```python
from build123d import *

# Parameters (mm, degrees)
F1_R     = 6.5
F1_R_2   = 5.5
F3_DEPTH = 3
F4_DEPTH = 1.5
F5_DEPTH = 0.6
F6_DEPTH = 1
F7_DEPTH = 1
F8_DEPTH = 1


# Not quite as in the source:
# - ends of sketch curves that miss each other by under 0.0002 mm in the source are joined
# - the dataset's text gives a spline's control points without its knots; the knots are read off the source's solid


with BuildPart() as f3:
    # F1 (on Front) → F3 (new body)
    with BuildSketch(Plane.XZ):
        with Locations((1.996e-07, 0.145563783)):
            Circle(F1_R)
        with Locations((1.996e-07, 0.145563783)):
            Circle(F1_R_2, mode=Mode.SUBTRACT)
    extrude(amount=-F3_DEPTH)

    # F0 (on Front) + F1 (on Front) → F4 (join)
    with BuildSketch(Plane.XZ):
        with BuildLine():
            add(Edge.make_bspline(
                [(-1.4633628161, -3.8408698747), (-0.8618942381, -4.0797628795), (1.7775925035, -4.2725148883), (2.1266039699, -2.4883414841), (2.1792066492, -0.8570773415), (2.1261946367, 0.7652860278), (1.8591945487, 1.4152828688), (2.1073079889, 1.4090746613), (2.1070261206, 1.5973545621), (1.8482611221, 1.6571502022), (1.9106924097, 2.0013449435), (1.883292753, 2.4559971082), (1.4530608962, 2.5796008165), (1.3486705812, 2.982608362), (0.9522813685, 3.1051443516), (0.6376593936, 3.1670181532), (0.4331394013, 3.4063180529), (0.6426984155, 3.8176132891), (0.3981993423, 4.2634916825), (-0.0062082347, 4.3047771669), (-0.3006353253, 4.2313929361), (-0.6271454426, 3.9609581822), (-0.5601436399, 3.6082200906), (-0.4158755178, 3.3585569408), (-0.6804152796, 3.1141950016), (-1.0068060059, 3.1249120402), (-1.1963426018, 2.8920399235), (-1.3913162215, 2.8683333491), (-1.3804892819, 2.6236576239), (-1.7077578499, 2.7520009173), (-1.8276300328, 2.3206081403), (-1.8540486856, 2.0110635487), (-1.8641412125, 1.6986764558), (-2.1169141262, 1.6232767981), (-2.0818952059, 1.4062115725), (-1.9001690611, 1.4703026422), (-2.1146422172, 0.8809803752), (-2.0979861646, 0.2234423606), (-2.2011740498, -0.523800053), (-2.1724225003, -1.2230030424), (-2.1779022447, -2.5473945892), (-1.9120269544, -3.4285716282), (-1.7403824301, -3.7308424346), (-1.4633628161, -3.8408698747)],
                knots=[0, 0, 0, 0, 0.0614284178, 0.105210304, 0.1528188952, 0.1998934744, 0.2260159491, 0.2394622475, 0.2521789794, 0.2685961982, 0.2887254165, 0.3121716538, 0.3345624104, 0.3566054098, 0.3791085644, 0.3997521347, 0.4178904262, 0.4412373911, 0.4652934844, 0.487296569, 0.5074239254, 0.5296841222, 0.5504706917, 0.5687295132, 0.5882529988, 0.6087082105, 0.6278548545, 0.642595893, 0.6569229468, 0.674176944, 0.6961346625, 0.7176137944, 0.736576695, 0.7535032789, 0.767308469, 0.7778501968, 0.8029343179, 0.8341377518, 0.8649078271, 0.8956216456, 0.9374997946, 0.9717077879, 1, 1, 1, 1], degree=3))
        make_face()
    with BuildSketch(Plane.XZ):
        with Locations((1.996e-07, 0.145563783)):
            Circle(F1_R_2)
    extrude(amount=-F4_DEPTH)

    # F1 (on Front) + F0 (on Front) → F5 (cut)
    with BuildSketch(Plane.XZ):
        with Locations((1.996e-07, 0.145563783)):
            Circle(F1_R_2)
    with BuildSketch(Plane.XZ):
        with BuildLine():
            add(Edge.make_bspline(
                [(-1.4633628161, -3.8408698747), (-0.8618942381, -4.0797628795), (1.7775925035, -4.2725148883), (2.1266039699, -2.4883414841), (2.1792066492, -0.8570773415), (2.1261946367, 0.7652860278), (1.8591945487, 1.4152828688), (2.1073079889, 1.4090746613), (2.1070261206, 1.5973545621), (1.8482611221, 1.6571502022), (1.9106924097, 2.0013449435), (1.883292753, 2.4559971082), (1.4530608962, 2.5796008165), (1.3486705812, 2.982608362), (0.9522813685, 3.1051443516), (0.6376593936, 3.1670181532), (0.4331394013, 3.4063180529), (0.6426984155, 3.8176132891), (0.3981993423, 4.2634916825), (-0.0062082347, 4.3047771669), (-0.3006353253, 4.2313929361), (-0.6271454426, 3.9609581822), (-0.5601436399, 3.6082200906), (-0.4158755178, 3.3585569408), (-0.6804152796, 3.1141950016), (-1.0068060059, 3.1249120402), (-1.1963426018, 2.8920399235), (-1.3913162215, 2.8683333491), (-1.3804892819, 2.6236576239), (-1.7077578499, 2.7520009173), (-1.8276300328, 2.3206081403), (-1.8540486856, 2.0110635487), (-1.8641412125, 1.6986764558), (-2.1169141262, 1.6232767981), (-2.0818952059, 1.4062115725), (-1.9001690611, 1.4703026422), (-2.1146422172, 0.8809803752), (-2.0979861646, 0.2234423606), (-2.2011740498, -0.523800053), (-2.1724225003, -1.2230030424), (-2.1779022447, -2.5473945892), (-1.9120269544, -3.4285716282), (-1.7403824301, -3.7308424346), (-1.4633628161, -3.8408698747)],
                knots=[0, 0, 0, 0, 0.0614284178, 0.105210304, 0.1528188952, 0.1998934744, 0.2260159491, 0.2394622475, 0.2521789794, 0.2685961982, 0.2887254165, 0.3121716538, 0.3345624104, 0.3566054098, 0.3791085644, 0.3997521347, 0.4178904262, 0.4412373911, 0.4652934844, 0.487296569, 0.5074239254, 0.5296841222, 0.5504706917, 0.5687295132, 0.5882529988, 0.6087082105, 0.6278548545, 0.642595893, 0.6569229468, 0.674176944, 0.6961346625, 0.7176137944, 0.736576695, 0.7535032789, 0.767308469, 0.7778501968, 0.8029343179, 0.8341377518, 0.8649078271, 0.8956216456, 0.9374997946, 0.9717077879, 1, 1, 1, 1], degree=3))
        make_face()
    extrude(amount=-F5_DEPTH, mode=Mode.SUBTRACT)

    # F2 (on face) → F6 (join)
    with BuildSketch(Plane.XZ):
        with BuildLine():
            ThreePointArc((-0.6012813019, -3.9545493796), (2.6071895589, -3.0335725809), (4, 0))
            ThreePointArc((4, 0), (3.9985637458, 0.1071819529), (3.9942560145, 0.2142869356))
            add(Edge.make_bspline(
                [(0.6696937898, 3.9435403165), (0.6582621326, 3.6561648877), (0.748660393, 2.9819733395), (1.5906344476, 1.8060597163), (2.343729672, 1.0651587443), (3.5468225291, 0.2060757034), (3.8886131662, 0.2055288721), (3.9942560145, 0.2142869356)],
                knots=[0, 0, 0, 0, 0.1914441273, 0.4252731611, 0.6392341909, 0.8752207587, 1, 1, 1, 1], degree=3))
            ThreePointArc((0.6696937898, 3.9435403165), (-2.3798948862, 3.2149806112), (-3.9672180841, 0.5110583855))
            add(Edge.make_bspline(
                [(-3.9672180841, 0.5110583855), (-3.2570424953, 0.3072051337), (-2.8281277347, 0.1183736874), (-1.7521563519, -0.7910134795), (-1.1021707585, -1.5327189765), (-0.7270922455, -2.8181587186), (-0.5608016797, -3.6356710711), (-0.6012813019, -3.9545493796)],
                knots=[0, 0, 0, 0, 0.2105751714, 0.4131601255, 0.5959388752, 0.8062823722, 1, 1, 1, 1], degree=3))
        make_face()
    extrude(amount=-F6_DEPTH)

    # F2 (on face) → F7 (join)
    with BuildSketch(Plane.XZ):
        with BuildLine():
            ThreePointArc((-4, -5.4666e-06), (-3.1915709466, -2.4111978128), (-1.0930678122, -3.8477529492))
            add(Edge.make_bspline(
                [(-4, -5.4666e-06), (-3.8428166733, -0.0460123585), (-3.5603914777, -0.133738653), (-3.2985794295, -0.2386569495), (-3.1472677408, -0.3246867621), (-2.9956539452, -0.4287257802), (-2.8222463482, -0.557104318), (-2.5840878529, -0.7485534177), (-2.2954985412, -1.0016010876), (-2.036026908, -1.2482860637), (-1.8381629968, -1.4634144564), (-1.6835113586, -1.6757370022), (-1.5516009911, -1.9240469669), (-1.4256566149, -2.248184411), (-1.3146225307, -2.6109466281), (-1.2146554645, -2.9978949757), (-1.1313238625, -3.3629451013), (-1.0901758206, -3.651388342), (-1.0894246902, -3.7951254649), (-1.0930678122, -3.8477529492)],
                knots=[0.0110273175, 0.0110273175, 0.0110273175, 0.0110273175, 0.0625, 0.125, 0.1875, 0.21875, 0.25, 0.3125, 0.375, 0.4375, 0.5, 0.5625, 0.625, 0.6875, 0.75, 0.8125, 0.875, 0.9375, 0.9857876166, 0.9857876166, 0.9857876166, 0.9857876166], degree=3))
        make_face()
    extrude(amount=-F7_DEPTH)

    # F2 (on face) → F8 (join)
    with BuildSketch(Plane.XZ):
        with BuildLine():
            add(Edge.make_bspline(
                [(1.1680500995, 3.8256503793), (1.1697995693, 3.7107206965), (1.1918189199, 3.5214057887), (1.2802032379, 3.2411969251), (1.4118748463, 2.9720045965), (1.5937127908, 2.679461535), (1.8023614597, 2.3919954972), (2.0179930746, 2.1262894096), (2.2181018419, 1.9032227167), (2.4259640622, 1.6986298437), (2.6643415193, 1.4905337309), (2.9597106264, 1.2554890784), (3.2786287368, 1.0236228812), (3.5292013722, 0.8637020638), (3.6951311872, 0.7741756792), (3.7886457426, 0.7328710188), (3.8426743367, 0.7168415355), (3.8851876888, 0.7098421735), (3.9097876849, 0.7094994811), (3.9362444503, 0.7113026549)],
                knots=[0.0276671484, 0.0276671484, 0.0276671484, 0.0276671484, 0.125, 0.1875, 0.25, 0.3125, 0.375, 0.4375, 0.5, 0.5625, 0.625, 0.6875, 0.75, 0.8125, 0.84375, 0.875, 0.90625, 0.9375, 0.9898649034, 0.9898649034, 0.9898649034, 0.9898649034], degree=3))
            ThreePointArc((3.9362444503, 0.7113026549), (2.989694007, 2.6573915302), (1.1680500995, 3.8256503793))
        make_face()
    extrude(amount=-F8_DEPTH)


solid = f3.part
```
Geometry check sheet. Reference: the model listing, model coordinates, mm. A direction names the side the tool comes from. Coordinates: 2 decimals unless noted, no trailing zeros. Order: outer loops, then holes, each group sorted by start corner. A loop starts at its lowest first (then second) coordinate and runs counter-clockwise, first axis right, second up.
Item 1: Scan lines: line 1 along Z through (x, y) = (0, 0.35); line 2 along Z through (x, y) = (3.5, 0.25); line 3 along Z through (x, y) = (0, 2.4). Record each from-to range of solid material in increasing order.
Item 2: Depth check by flat-ended pin: pin 1 (1 mm diameter, centred on x = -2.5, y = 0.5, fed in from -Z). Enter the tip coordinate at first touch or a pass-through.
Item 3: Section check D-D (y = 0.8). Enter the section's corners in (x, z), plus the area to 3 significant figures.
Item 4: Section check C-C (x = 4.75). Enter the section's corners in (y, z), plus the area to 3 significant figures.
Item 5: Section check A-A (x = 0). Enter the section's corners in (y, z), plus the area to 3 significant figures.
Item 6: Tool access check on faces 1 (the flat face through (0, 0, 0)), 2 (the flat face through (0, 1.5, 0)), 3 (the cylindrical face through (3.01, 0.296, 2.634)). Record the directions out of +Z, -Z, +X, -X, +Y, -Y that give a thin tool (end or side, any length) a straight path to the whole face; none if there is none.
Item 7: Mould release check, pull along X, two halves, no side actions. Record for faces 4 (the cylindrical face through (-1.192, 2.24, -5.224)), 5 (the cylindrical face through (-1.4, 1.5, -6.2)), 6 (the flat face through (-5, 3, 3)): released by +X, released by -X, zero draft, split by the parting line, or undercut.
Item 8: Section check B-B (y = 2.7). Enter the section's corners in (x, z).
Check sheet entries:
1. line 1: z = -6.35 to -5.35, -4 to 4, 5.65 to 6.65
1. line 2: z = -5.33 to -4.1, -1.94 to 0.31, 0.88 to 1.94, 4.39 to 5.62
1. line 3: z = -6.35 to -5.35, 5.65 to 6.65
2. pin 1: stops at z = -6.04
3. outline: circle Ø13 at (0, 0.15)
3. area: 133 mm2
4. outline: (0, -4.29) - (3, -4.29) - (3, -2.63) - (1.5, -2.63) - (1.5, 2.92) - (3, 2.92) - (3, 4.58) - (0, 4.58) - (0, 2.92) - (0.6, 2.92) - (0.6, -2.63) - (0, -2.63) - close
4. area: 15.0 mm2
5. outline: (0, -6.35) - (3, -6.35) - (3, -5.35) - (1.5, -5.35) - (1.5, 5.65) - (3, 5.65) - (3, 6.65) - (0, 6.65) - (0, 5.65) - (0.6, 5.65) - (0.6, 4) - (0, 4) - (0, -4) - (0.6, -4) - (0.6, -5.35) - (0, -5.35) - close
5. area: 20.7 mm2
6. face 1: +Z, -Z, +X, -X, -Y
6. face 2: +Y
6. face 3: -Y
7. face 4: undercut
7. face 5: split by the parting line
7. face 6: zero draft
8. outline: circle Ø13 at (0, 0.15); hole circle Ø11 at (0, 0.15)
